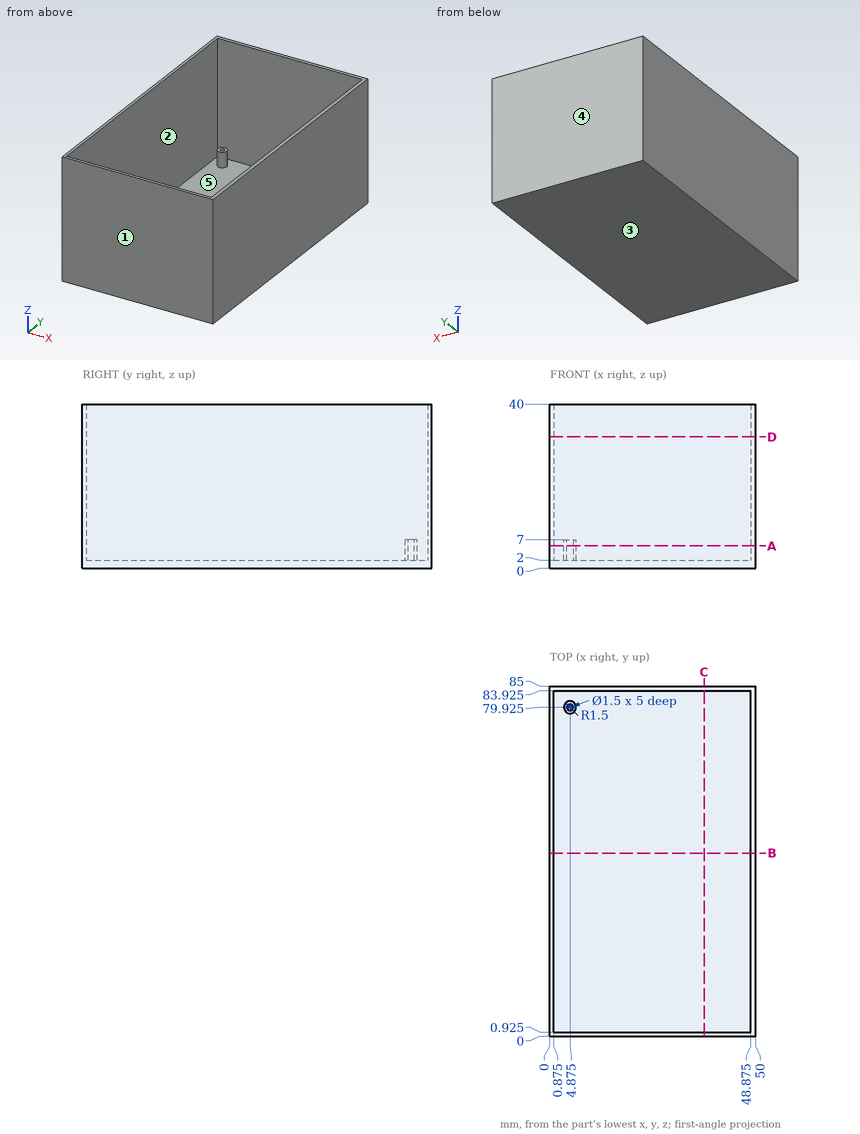
Here's the drawing with two shaded views (mm, measured from the low corner). I have some questions. A direction names the side the tool comes from. Round coordinates to 2 decimals unless told otherwise and drop trailing zeros. Order: outer loops, then holes, each group sorted by start corner. A loop starts at its lowest first (then second) coordinate and runs counter-clockwise, first axis right, second up. Notation, with made-up numbers: (25, 88) -> (63, 88) arc R31 cw to (63, 124) -> close; hole circle Ø8 at (34, 60). An arc over 180 degrees is marked (long way). Return JSON: item names as keys, results as strings.
Q1. For pin 1 Ø2 at (x, y) = (43.5, 72) entering from +Z; pin 2 Ø1.5 at (x, y) = (5.5, 80) entering from +Z, each with a flat end and sliding along its axis, tell me the tip position at first contact or that it passes through.
Filled sheet:
{"pin 1": "stops at z = 2", "pin 2": "stops at z = 7"}
Q2. If we mould it in two halves opening along Y, with no side actions, what happens to the marked faces 1, 2 and 3? For each: released by +Y, released by -Y, zero draft, split by the parting line, or undercut.
Filled sheet:
{"face 1": "released by -Y", "face 2": "undercut", "face 3": "zero draft"}
Q3. If we section it at D-D on z = 32: List the corners of the cut face in (x, y) for me (1 decimal).
Filled sheet:
{"outline": "(0, 0) -> (50, 0) -> (50, 85) -> (0, 85) -> close; hole (0.9, 0.9) -> (48.9, 0.9) -> (48.9, 83.9) -> (0.9, 83.9) -> close"}
Q4. If we section it at B-B on y = 44.5: List the corners of the cut face in (x, z) for me (1 decimal).
Filled sheet:
{"outline": "(0, 0) -> (50, 0) -> (50, 40) -> (48.9, 40) -> (48.9, 2) -> (0.9, 2) -> (0.9, 40) -> (0, 40) -> close"}
Q5. Which directions (+Z, -Z, +X, -X, +Y, -Y) give clear straight access to the entire face, cutting with the end or side of a thin tool? Please do the marked faces 4 and 5.
Filled sheet:
{"face 4": "+Z, -Z, +X, -X, +Y", "face 5": "+Z"}
Q6. I need wall thicknesses on line 1 along Y through (x, z) = (45, 6) (1 decimal); line 2 along X through (y, z) = (27, 17) (1 decimal); line 3 along Z through (x, y) = (30.5, 19). Which ranges of each line are inside material? Lowest first, please. Write a range as from..to.
Filled sheet:
{"line 1": "y = 0..0.9, 83.9..85", "line 2": "x = 0..0.9, 48.9..50", "line 3": "z = 0..2"}
Q7. If we section it at C-C on x = 37.5: List the corners of the cut face in (y, z) for me (1 decimal).
Filled sheet:
{"outline": "(0, 0) -> (85, 0) -> (85, 40) -> (83.9, 40) -> (83.9, 2) -> (0.9, 2) -> (0.9, 40) -> (0, 40) -> close"}
Q8. If we section it at A-A on z = 5.5: Give the number of separate pieces and of enclosed holes in the cut face.
Filled sheet:
{"separate pieces": "2", "enclosed holes": "2"}
